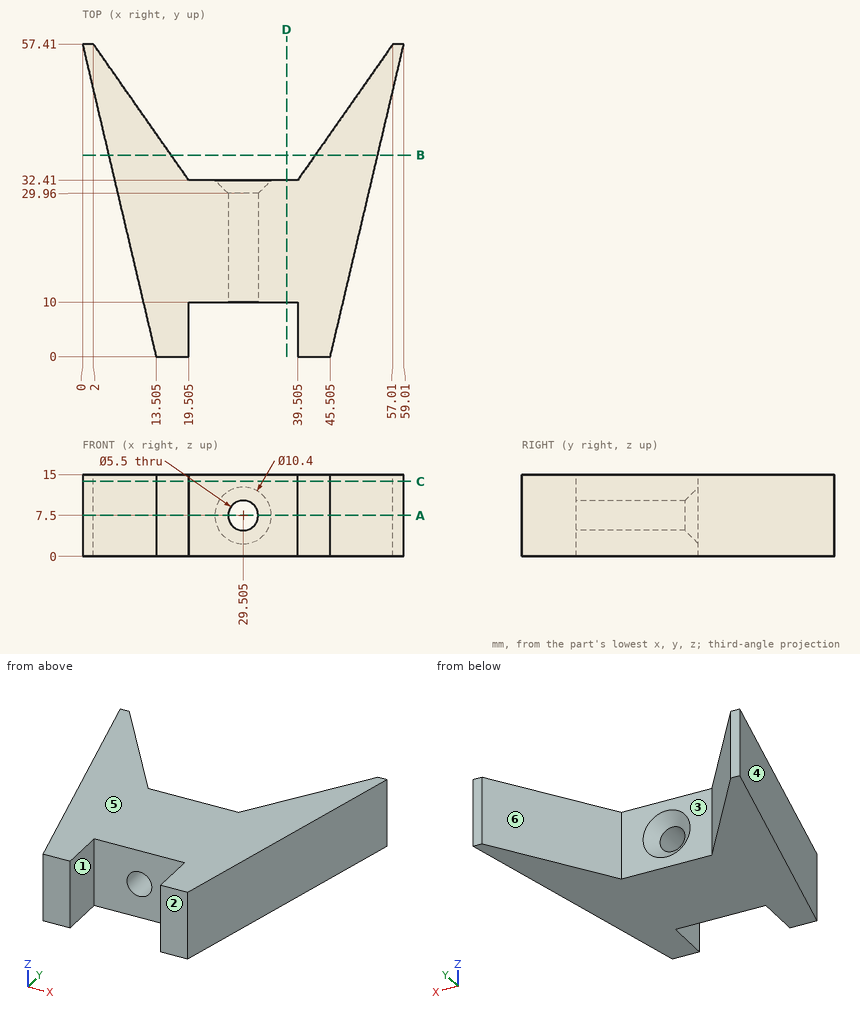
The drawing under review shows one solid part. Ordinate dimensions are in mm from its lowest x, y, z. A direction names the side the tool comes from. Round coordinates to 2 decimals unless told otherwise and drop trailing zeros. Loops run counter-clockwise (first coordinate to the right, second up) from the corner with the lowest first, then second, coordinate; pieces in that order, holes last. Notation, with made-up numbers: (30.5, 52) - (82.5, 52) arc R27 cw to (82.5, 78) - close; hole circle Ø11 at (8.25, -10). An arc over 180 degrees is marked (long way). One line per item, written item: value. Start each with the question number.
1) Insertion check: pin 1 Ø5 at (y, z) = (4, 4) entering from -X; pin 2 Ø1.5 at (x, z) = (21, 11) entering from -Y; pin 3 Ø1 at (y, z) = (43, 6.5) entering from +X; pin 4 Ø5 at (x, z) = (29.51, 7.5) entering from -Y. Each pin has a flat end and moves straight along its axis. Give the tip position at first contact, or say it passes through.
2) Consider section A-A on z = 7.5. Give the boundary of the cut face in (x, y) (1 decimal), then the cut area to 3 significant figures.
3) Consider section C-C on z = 13.75. Give the boundary of the cut face in (x, y) (1 decimal).
4) To check wall thickness, follow L1, parallel to Y at x = 38, z = 11; L2, parallel to X at y = 8.5, z = 11.75 (1 decimal); L3, parallel to X at y = 34.5, z = 10.75. State the ranges of each line that lie inside material, in increasing order. Write a range as from..to.
5) Draft analysis for pull direction X (two halves, no side actions). For the marked faces 4, 5 and 6, state which applies: +X half, -X half, draft (parallel to the pull), parting line (faces both ways), or undercut.
6) For the marked faces 1, 2 and 3, list the 3-axis set-ups (+Z, -Z, +X, -X, +Y, -Y) from which the entire face can be reached by the end or side of a thin tool; tool diameter is ignored.
7) Consider section B-B on y = 37. Give the boundary of the cut face in (x, z), then the cut area to 3 significant figures.
8) Consider section D-D on x = 37.5. Give the boundary of the cut face in (y, z).
Reported:
1. pin 1: stops at x = 11.98
1. pin 2: stops at y = 10
1. pin 3: stops at x = 55.74
1. pin 4: passes through
2. outline: (0, 57.4) - (13.5, 0) - (19.5, 0) - (19.5, 10) - (26.8, 10) - (26.8, 30) - (24.3, 32.4) - (19.5, 32.4) - (2, 57.4) - close; (32.3, 10) - (39.5, 10) - (39.5, 0) - (45.5, 0) - (59, 57.4) - (57, 57.4) - (39.5, 32.4) - (34.7, 32.4) - (32.3, 30) - close
2. area: 1,350 mm^2
3. outline: (0, 57.4) - (13.5, 0) - (19.5, 0) - (19.5, 10) - (39.5, 10) - (39.5, 0) - (45.5, 0) - (59, 57.4) - (57, 57.4) - (39.5, 32.4) - (19.5, 32.4) - (2, 57.4) - close
4. L1: y = 10..32.41
4. L2: x = 11.5..19.5, 39.5..47.5
4. L3: x = 5.39..18.04, 40.97..53.62
5. face 4: -X half
5. face 5: draft
5. face 6: undercut
6. face 1: +Z, -Z, -Y
6. face 2: +Z, -Z, +X, -X, -Y
6. face 3: +Z, -Z, +Y
7. outline: (4.8, 0) - (16.29, 0) - (16.29, 15) - (4.8, 15) - close; (42.72, 0) - (54.21, 0) - (54.21, 15) - (42.72, 15) - close
7. area: 345 mm^2
8. outline: (10, 0) - (32.41, 0) - (32.41, 15) - (10, 15) - close
